Read the model definition and answer for the solid it produces. Units are mm, in the model's axes. A direction names the side the tool comes from. Coordinates: 2 decimals unless noted, no trailing zeros. Write each loop counter-clockwise with the first axis right and the second up, starting at its lowest first coordinate (ties: lowest second). Pieces come first, ordered by that corner, then holes. Notation, with made-up numbers: (7.25, 29.25) -> (26.25, 29.25) arc R21 ccw to (26.25, 37.25) -> close; hole circle Ø5 at (41, 73). An arc over 180 degrees is marked (long way). Write item = value, one per line. Start each with the question number.
1) A tool of negligible diameter and unlimited length cuts with its end or side. For faces 1 (the face through (-14.3, -60.4, -10)), 2 (the face through (-20, 27.89, 7.57)), 3 (the face through (-11, -36, 2.5)), from which of +Z, -Z, +X, -X, +Y, -Y can it reach the whole face along a straight path? Write none if from no direction.
2) For a pull along Y with two mould halves and no side action, classify faces 4 (the face through (-60.15, 59.99, 11.23)), 5 (the face through (59.99, -60.15, 11.27)), 6 (the face through (-14.155, -31.263, 7.57)), 7 (the face through (-53.19, 54.54, 0.18)) as released by +Y, released by -Y, zero draft, split by the parting line, or undercut.
3) Flat-ended cylindrical pins translate along their axes: pin 1 Ø3 at (y, z) = (-44.5, 8) entering from +X; pin 2 Ø4 at (y, z) = (45.5, 1.5) entering from -X; pin 3 Ø1.5 at (x, z) = (47.5, -2) entering from -Y; pin 4 Ø6.5 at (x, y) = (55.5, 55.5) entering from -Z. Find the tip coordinate at first contact, or state that the pin passes through.
4) Section A-A (z = -3) is taken. Count the separate pieces of the cut face and the enclosed holes in it, plus the area to 3 significant figures.
5) Section D-D (x = -24) is taken. Determine the outline of the cut face in (y, z).
6) Find the intervals of material crossed by line 1 along Y through (x, z) = (0, -7.25); line 2 along X through (y, z) = (7, 9.5) (3 decimals); line 3 along Y through (x, z) = (0, 5.25), in increasing order. Write a range as from..to.
from build123d import *

# Parameters (mm, degrees)
F0_W     = 126
F0_H     = 126
F1_DEPTH = 12.5
F6_R     = 60
F6_R_2   = 20
F6_R_3   = 2.5
F7_DEPTH = 25.001
F3_DEPTH = 10
F4_W     = 126
F4_H     = 126
F4_R     = 3.75
F4_R_2   = 61.5
F8_DEPTH = 10
F5_R     = 10


with BuildPart() as f1:
    # F0 (on Top) → F1 (new body, symmetric)
    with BuildSketch(Plane.XY):
        Rectangle(F0_W, F0_H)
    extrude(amount=F1_DEPTH, both=True)

    # F6 (on face) → F7 (cut, through all)
    with BuildSketch(Plane.XY.offset(12.5)):
        Circle(F6_R)
        Circle(F6_R_2, mode=Mode.SUBTRACT)
        with Locations((55.5, -55.5)):
            Circle(F6_R_3)
        with Locations((-55.5, -55.5)):
            Circle(F6_R_3)
        with Locations((-55.5, 55.5)):
            Circle(F6_R_3)
        with Locations((55.5, 55.5)):
            Circle(F6_R_3)
    extrude(amount=-F7_DEPTH, mode=Mode.SUBTRACT)

    # F2 (on face) → F3 (join)
    with BuildSketch(Plane.XY.offset(12.5)):
        with BuildLine():
            Line((6.416974, 18.942609), (-47.160816, 37.092552))
            ThreePointArc((-47.160816, 37.092552), (-48.731962, 35.002798), (-50.210577, 32.846582))
            Line((-50.210577, 32.846582), (-7.716628, 18.451386))
            ThreePointArc((-7.716628, 18.451386), (-0.694694, 19.987931), (6.416974, 18.942609))
        make_face()
        with BuildLine():
            ThreePointArc((-8.542685, -59.388741), (-5.947332, -59.704516), (-3.340686, -59.906926))
            Line((-3.340686, -59.906926), (-12.121055, -15.908489))
            ThreePointArc((-12.121055, -15.908489), (-16.962709, -10.595589), (-19.613268, -3.914042))
            Line((-19.613268, -3.914042), (-8.542685, -59.388741))
        make_face()
        with BuildLine():
            ThreePointArc((55.703501, 22.296188), (54.679293, 24.701718), (53.551263, 27.060344))
            Line((53.551263, 27.060344), (19.837683, -2.542897))
            ThreePointArc((19.837683, -2.542897), (17.657403, -9.392343), (13.196294, -15.028567))
            Line((13.196294, -15.028567), (55.703501, 22.296188))
        make_face()
    extrude(amount=-F3_DEPTH)

    # F4 (on Top) → F8 (cut, symmetric)
    with BuildSketch(Plane.XY):
        Rectangle(F4_W, F4_H)
        with Locations((-55.5, -55.5)):
            Circle(F4_R, mode=Mode.SUBTRACT)
        with Locations((55.5, -55.5)):
            Circle(F4_R, mode=Mode.SUBTRACT)
        with Locations((-55.5, 55.5)):
            Circle(F4_R, mode=Mode.SUBTRACT)
        Circle(F4_R_2, mode=Mode.SUBTRACT)
        with Locations((55.5, 55.5)):
            Circle(F4_R, mode=Mode.SUBTRACT)
    extrude(amount=F8_DEPTH, both=True, mode=Mode.SUBTRACT)

    # F5
    f5_edges = [f1.edges().sort_by_distance(p)[0] for p in [
        (63, 63, -11.25),
        (63, 63, 11.25),
        (-63, 63, -11.25),
        (-63, 63, 11.25),
        (-63, -63, -11.25),
        (-63, -63, 11.25),
        (63, -63, -11.25),
        (63, -63, 11.25),
    ]]
    fillet(f5_edges, radius=F5_R)


solid = f1.part
Answer key:
q1.face_1 = none
q1.face_2 = +Z, -Z
q1.face_3 = -Z
q2.face_4 = released by +Y
q2.face_5 = released by -Y
q2.face_6 = undercut
q2.face_7 = undercut
q3.pin_1 = 43.97
q3.pin_2 = -43.47
q3.pin_3 = -39.96
q3.pin_4 = -12.5
q4.separate_pieces = 6
q4.enclosed_holes = 5
q4.area = 1,930 mm^2
q5.outline = (-63, -12.5) -> (-54.99, -12.5) -> (-54.99, 12.5) -> (-63, 12.5) -> (-63, 10) -> (-56.62, 10) -> (-56.62, -10) -> (-63, -10) -> close; (23.97, 2.5) -> (29.25, 2.5) -> (29.25, 12.5) -> (23.97, 12.5) -> close; (54.99, -12.5) -> (63, -12.5) -> (63, -10) -> (56.62, -10) -> (56.62, 10) -> (63, 10) -> (63, 12.5) -> (54.99, 12.5) -> close
q6.line_1 = -61.5..-60, -20..20, 60..61.5
q6.line_2 = -61.1..-59.59, -18.735..18.735, 30.706..38.283, 59.59..61.1
q6.line_3 = -61.5..-60, -20..21.12, 60..61.5
